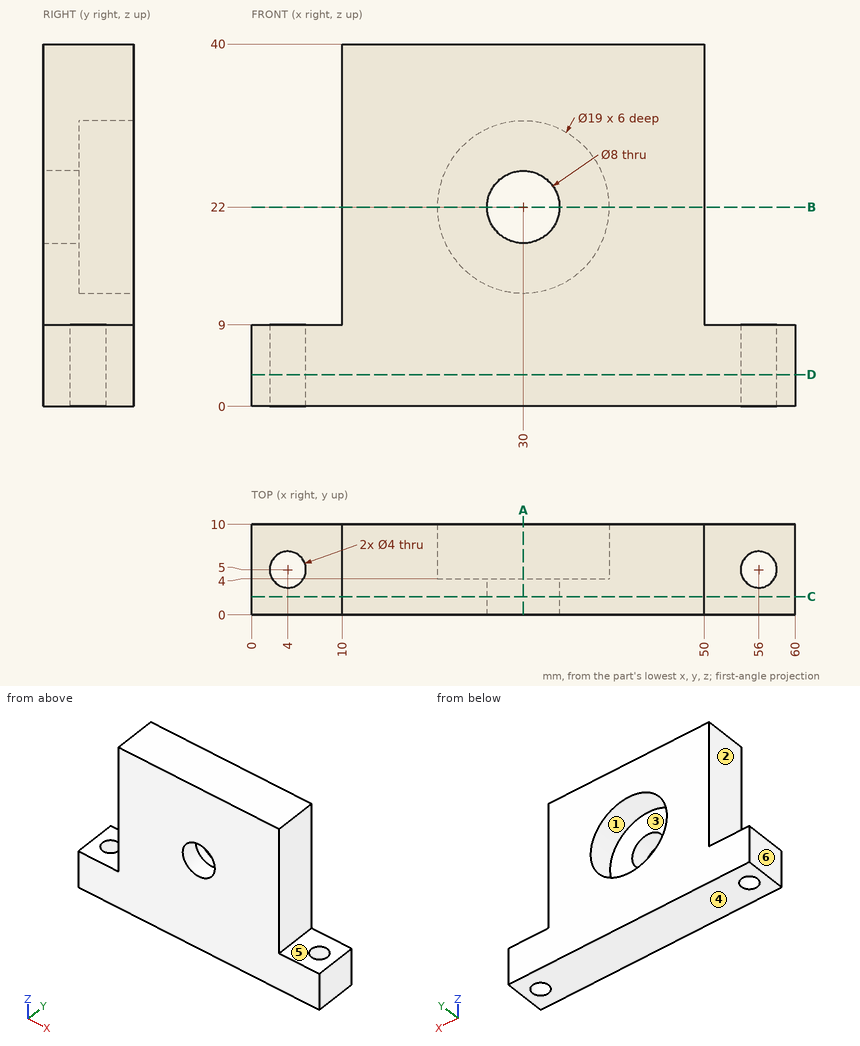
Part print with two shaded views. Sizes in mm from the minimum x, y, z corner. A direction names the side the tool comes from. Round coordinates to 2 decimals unless told otherwise and drop trailing zeros. Loops run counter-clockwise (first coordinate to the right, second up) from the corner with the lowest first, then second, coordinate; pieces in that order, holes last. Notation, with made-up numbers: (87, 58) - (107, 58) arc R23 cw to (107, 81) - close; hole circle Ø3 at (-31.5, 19). An arc over 180 degrees is marked (long way). Answer as a JSON object with one key per item and string values.
Item 1: Band-saw the part on B-B on z = 22. List the corners of the cut face in (x, y), plus the area to 3 significant figures.
Output:
{"outline": "(10, 0) - (26, 0) - (26, 4) - (20.5, 4) - (20.5, 10) - (10, 10) - close; (34, 0) - (50, 0) - (50, 10) - (39.5, 10) - (39.5, 4) - (34, 4) - close", "area": "254 mm2"}
Item 2: Pin check, flat tips, straight feed: pin 1 (3 mm diameter, centred on x = 5.5, y = 5.5, fed in from +Z); pin 2 (2 mm diameter, centred on y = 3, z = 12.5, fed in from +X). Stop position of each tip, or through.
Output:
{"pin 1": "z = 9", "pin 2": "x = 50"}
Item 3: Pull direction X, two halves, no side cores. Call the marked faces 1, 2, 3 and 4: pulls with the +X half, pulls with the -X half, needs draft (parallel to the pull), parting line crosses it, or undercut.
Output:
{"face 1": "undercut", "face 2": "pulls with the -X half", "face 3": "undercut", "face 4": "needs draft"}
Item 4: Wall check: L1, parallel to X at y = 5, z = 7; L2, parallel to X at y = 6.7, z = 22; L3, parallel to Y at x = 56, z = 3.5. Give the ranges that are in metal, low to high.
Output:
{"L1": "0 to 2, 6 to 54, 58 to 60", "L2": "10 to 20.5, 39.5 to 50", "L3": "0 to 3, 7 to 10"}
Item 5: Band-saw the part on A-A on x = 30. List the corners of the cut face in (y, z).
Output:
{"outline": "(0, 0) - (10, 0) - (10, 12.5) - (4, 12.5) - (4, 18) - (0, 18) - close; (0, 26) - (4, 26) - (4, 31.5) - (10, 31.5) - (10, 40) - (0, 40) - close"}
Item 6: Tool access for the marked faces 5 and 6: list every direction of +Z, -Z, +X, -X, +Y, -Y with a clear straight run to the whole face (end or side of a thin tool).
Output:
{"face 5": "+Z, +X, +Y, -Y", "face 6": "+Z, -Z, -X, +Y, -Y"}
Item 7: Band-saw the part on D-D on z = 3.5. List the corners of the cut face in (x, y).
Output:
{"outline": "(0, 0) - (60, 0) - (60, 10) - (0, 10) - close; hole circle Ø4 at (4, 5); hole circle Ø4 at (56, 5)"}
Item 8: Band-saw the part on C-C on y = 2. List the corners of the cut face in (x, z), plus the area to 3 significant figures.
Output:
{"outline": "(0, 0) - (60, 0) - (60, 9) - (50, 9) - (50, 40) - (10, 40) - (10, 9) - (0, 9) - close; hole circle Ø8 at (30, 22)", "area": "1,730 mm2"}
